Design review of the part built by this model. Coordinates are the model's own, in mm. Face numbers are marked on the shaded views. Give positions to 0.01 mm unless a question says otherwise; leave off trailing zeros. Order: outer loops, then holes, each group sorted by start corner. A loop starts at its lowest first (then second) coordinate and runs counter-clockwise, first axis right, second up. Notation, with made-up numbers: (-29, 25) -> (15, 25) arc R19 cw to (15, 59) -> close; hole circle Ø5 at (69, 62.25). An arc over 180 degrees is marked (long way). One line per item, written item: value.
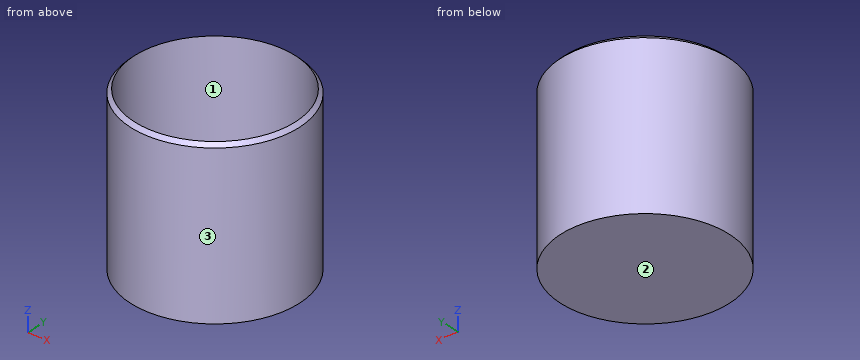
from build123d import *

# Parameters (mm, degrees)
F0_R     = 57.7707410697
F1_DEPTH = 114.3
F2_T     = -2.54


# Not quite as in the source:
# - a fillet or chamfer that OpenCascade refuses, or shapes differently, is made with other operations: its cross-section is extruded or revolved along the edge and cut away or added
# - the program builds the solid bodies; features that only make, move or delete a surface that nothing else refers to are left out


with BuildPart() as f1:
    # F0 (on Top) → F1 (new body)
    with BuildSketch(Plane.XY):
        Circle(F0_R)
    extrude(amount=-F1_DEPTH)

    # F2
    f2_openings = [f1.faces().sort_by_distance(p)[0] for p in [
        (0, 0, 0),
    ]]
    offset(amount=F2_T, openings=f2_openings)

    # F3: chamfer of 5.08 on 1 edges, made by hand

    # F3_s1 → F3_t2 (revolve, cut)
    with BuildSketch(Plane.XZ):
        Polygon((57.7707410697, -5.08), (52.6907410697, 0), (57.7707410697, 0), align=None)
    revolve(axis=Axis((0, 0, 0), (0, 0, 1)), mode=Mode.SUBTRACT)


solid = f1.part
Item 1: Clearance check with flat-ended pins moving along their axes: P1, Ø3, axis at x = -19.5, y = 7.5, coming from the +Z side; P2, Ø10, axis at y = 23.5, z = -59.5, coming from the +X side; P3, Ø6, axis at x = 15, z = -69.5, coming from the -Y side. State where each tip first meets the part, or that it passes through.
Returned:
P1: z = -111.76
P2: x = 54.73
P3: y = -56.51
Item 2: To check wall thickness, follow line 1 along Y through (x, z) = (0, -47); line 2 along Z through (x, y) = (-22, -5.5); line 3 along Y through (x, z) = (4, -12.5). State the ranges of each line that lie inside material, in increasing order. Write a range as from..to.
Returned:
line 1: -57.77..-55.23, 55.23..57.77
line 2: -114.3..-111.76
line 3: -57.63..-55.09, 55.09..57.63
Item 3: Add section B-B on z = -44. Give the boundary of the cut face in (x, y), plus the area to 3 significant figures.
Returned:
outline: circle Ø115.54 at (0, 0); hole circle Ø110.46 at (0, 0)
area: 902 mm²
Item 4: Add section A-A on x = 0. Give the boundary of the cut face in (y, z).
Returned:
outline: (-57.77, -114.3) -> (57.77, -114.3) -> (57.77, -5.08) -> (55.23, -2.54) -> (55.23, -111.76) -> (-55.23, -111.76) -> (-55.23, -2.54) -> (-57.77, -5.08) -> close
Item 5: Draft analysis for pull direction X (two halves, no side actions). For the marked faces 1, 2 and 3, state which applies: pulls with the +X half, pulls with the -X half, needs draft (parallel to the pull), parting line crosses it, or undercut.
Returned:
face 1: undercut
face 2: needs draft
face 3: parting line crosses it
